```python
from build123d import *

# Parameters (mm, degrees)
PAD013_DEPTH    = 6
POCKET007_DEPTH = 78.001
SKETCH019_W     = 2
SKETCH019_H     = 5.3
POCKET008_DEPTH = 6.001
SKETCH020_W     = 11.115
SKETCH020_H     = 2
POCKET009_DEPTH = 2
SKETCH021_R     = 1.5
POCKET010_DEPTH = 72.001
SKETCH022_R     = 1.5
POCKET011_DEPTH = 65.001


with BuildPart() as part:
    # Sketch017 → Pad013 (new body)
    with BuildSketch(Plane.XZ):
        with BuildLine():
            Line((-15.9, 6), (-15.9, 29.15))
            ThreePointArc((-1.8, 29.15), (-8.85, 36.2), (-15.9, 29.15))
            Line((-1.8, 0), (-1.8, 29.15))
            Line((9.315, 0), (-1.8, 0))
            Line((9.315, 0), (9.315, 13))
            Line((9.315, 13), (16.815, 13))
            Line((16.815, 13), (16.815, 39.5))
            Line((16.815, 39.5), (9.315, 39.5))
            Line((9.315, 39.5), (9.315, 78))
            Line((9.315, 78), (-15.9, 78))
            Line((-15.9, 78), (-15.9, 45.5))
            Line((-23.4, 45.5), (-15.9, 45.5))
            Line((-23.4, 6), (-23.4, 45.5))
            Line((-23.4, 6), (-15.9, 6))
        make_face()
    extrude(amount=PAD013_DEPTH)

    # Sketch018 (on Face5 of Pad013) → Pocket007 (cut, through all)
    with BuildSketch(Plane(origin=(0, 0, 0), x_dir=(1, 0, 0), z_dir=(0, 0, -1))):
        Polygon((-1.8, 6), (3.7575, 2), (9.315, 6), align=None)
    extrude(amount=-POCKET007_DEPTH, mode=Mode.SUBTRACT)

    # Sketch019 (on Face5 of Pocket007) → Pocket008 (cut, through all)
    with BuildSketch(Plane.XZ.offset(6)):
        with BuildLine():
            Line((-8.8500001165, 36.2), (-1.8, 36.2))
            Line((-1.8, 36.2), (-1.8, 34.2))
            Line((-1.8, 34.2), (-3.9306504495, 34.2))
            ThreePointArc((-3.9306504495, 34.2), (-6.1948164445, 35.6808881698), (-8.8500001165, 36.2))
        make_face()
        with Locations((10.315, 36.85)):
            Rectangle(SKETCH019_W, SKETCH019_H)
    extrude(amount=-POCKET008_DEPTH, mode=Mode.SUBTRACT)

    # Sketch020 (on Face4 of Pocket008) → Pocket009 (cut)
    with BuildSketch(Plane(origin=(0, 0, 0), x_dir=(1, 0, 0), z_dir=(0, 1, 0))):
        with Locations((3.7575, -35.2)):
            Rectangle(SKETCH020_W, SKETCH020_H)
    extrude(amount=-POCKET009_DEPTH, mode=Mode.SUBTRACT)

    # Sketch021 (on Face1 of Pocket009) → Pocket010 (cut, through all)
    with BuildSketch(Plane(origin=(0, 0, 6), x_dir=(1, 0, 0), z_dir=(0, 0, -1))):
        with Locations((-19.65, 3)):
            Circle(SKETCH021_R)
    extrude(amount=-POCKET010_DEPTH, mode=Mode.SUBTRACT)

    # Sketch022 (on Face31 of Pocket010) → Pocket011 (cut, through all)
    with BuildSketch(Plane(origin=(0, 0, 13), x_dir=(1, 0, 0), z_dir=(0, 0, -1))):
        with Locations((13.065, 3)):
            Circle(SKETCH022_R)
    extrude(amount=-POCKET011_DEPTH, mode=Mode.SUBTRACT)


with BuildPart() as part_1:
    # Body003 placement: moved
    add(part.part.moved(Location((0, -70, 0))))


solid = part_1.part
```
Geometry: final body of the model. Coordinates: model frame, mm. A direction names the side the tool comes from. Round coordinates to 2 decimals unless told otherwise and drop trailing zeros. Order: outer loops, then holes, each group sorted by start corner. A loop starts at its lowest first (then second) coordinate and runs counter-clockwise, first axis right, second up. Notation, with made-up numbers: M 50,13.5 L 62,13.5 A7 cw 62,23.5 Z; hole C 59,-13.5 d2. An arc over 180 degrees is marked long. Use one line per item in the form item = value. Start each with the question number.
Q1. Cut plane B-B (z = 20). Count the separate pieces of the cut face and the enclosed holes in it, and give its area (3 significant figures).
Q2. Material intervals for line 1 (X direction, y = -71.75, z = 20) (3 decimals); line 2 (X direction, y = -73, z = 30) (3 decimals); line 3 (Z direction, x = 9, y = -71.5), sorted ascending. Write a range as [from, to].
Q3. Pin query (flat end, axial travel): pin 1 Ø1 at (x, z) = (0, 35.5) entering from +Y; pin 2 Ø3 at (x, z) = (1.5, 53.5) entering from -Y; pin 3 Ø1 at (y, z) = (-74, 64) entering from +X (3 decimals). Return the tip coordinate at first contact, or that it passes through.
Q4. Mould query, pull axis X, two halves, no side actions, for faces 5 (the face through (13, -76, 26)), 6 (the face through (0.94, -74.03, 38.45)), 7 (the face through (-15.9, -73, 62)). Classes: +X half, -X half, draft (parallel to the pull), parting line (faces both ways), or undercut.
Q5. Access query for faces 1 (the face through (6.497, -73.972, 38.454)), 2 (the face through (3.6, -71.7, 34.2)), 3 (the face through (15, -73, 13)), 4 (the face through (-13.78, -72.96, 34.19)). Directions: +Z, -Z, +X, -X, +Y, -Y. A direction counts if a zero-diameter tool reaches every point of the face in a straight line with its end or side. Return the directions, or none.
Q6. Cut plane A-A (x = -19.65). Return loops of the section in (y, z), and give its area (4 significant figures).
Geometry results:
q1.separate_pieces = 2
q1.enclosed_holes = 2
q1.area = 120 mm^2
q2.line_1 = [-23.4, -20.479], [-18.821, -15.9], [-1.8, 12.236], [13.894, 16.815]
q2.line_2 = [-23.4, -21.15], [-18.15, -15.849], [-1.851, 2.368], [5.147, 11.565], [14.565, 16.815]
q2.line_3 = [0, 34.2], [36.2, 78]
q3.pin_1 = -72
q3.pin_2 = -74.7
q3.pin_3 = 9.315
q4.face_5 = draft
q4.face_6 = undercut
q4.face_7 = -X half
q5.face_1 = +Z, -Z, -Y
q5.face_2 = +Y
q5.face_3 = -Z, +X, +Y, -Y
q5.face_4 = -Z, +Y, -Y
q6.outline = M -76,6 L -74.5,6 L -74.5,45.5 L -76,45.5 Z; M -71.5,6 L -70,6 L -70,45.5 L -71.5,45.5 Z
q6.area = 118.5 mm^2
